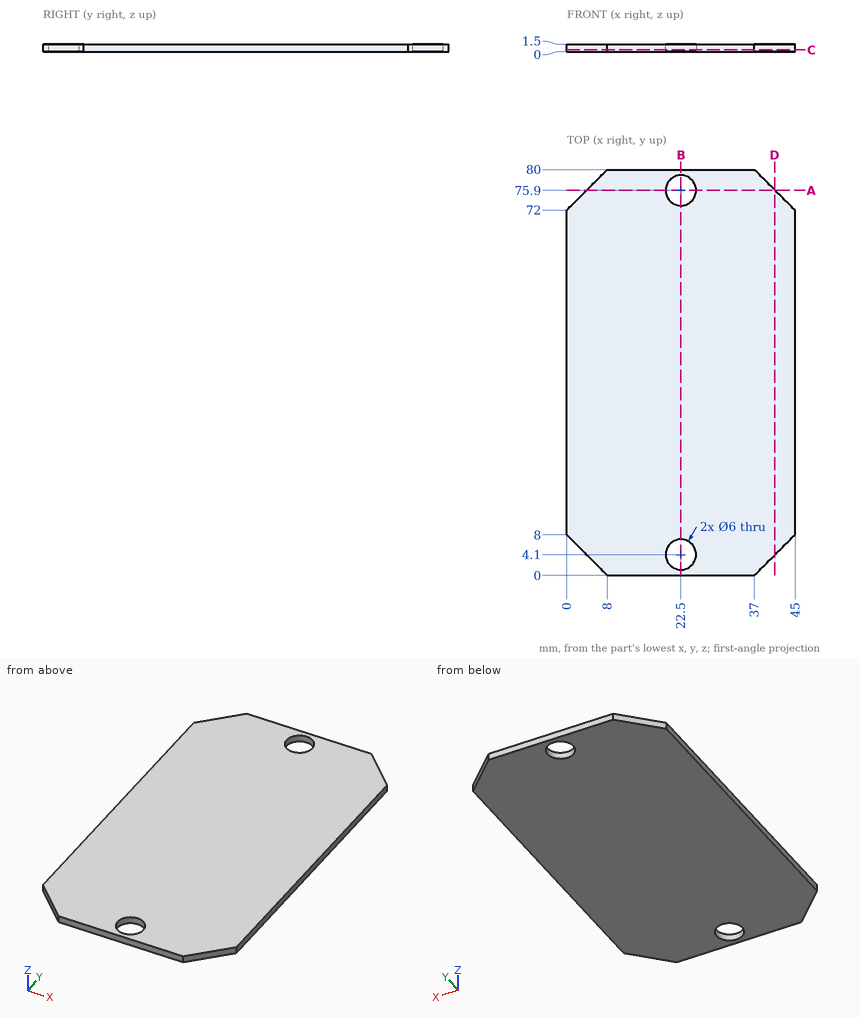
Answer from the drawing. Dimensions are ordinates in mm from the lowest x, y and z of the part. Round coordinates to 2 decimals unless told otherwise and drop trailing zeros. Order: outer loops, then holes, each group sorted by start corner. A loop starts at its lowest first (then second) coordinate and runs counter-clockwise, first axis right, second up.
1) The part is cut by section B-B on x = 22.5. Write down the section's boundary in (y, z).
2) Straight lines are drawn through the part: L1, parallel to Y at x = 22.5, z = 1.1; L2, parallel to Y at x = 20.5, z = 0.5; L3, parallel to X at y = 76.5, z = 0.7. For each, find the intervals that lie inside material, in ascending order.
3) The part is cut by section D-D on x = 41. Write down the section's boundary in (y, z), plus the area to 3 significant figures.
4) The part is cut by section C-C on z = 0.35. Write down the section's boundary in (x, y).
5) The part is cut by section A-A on y = 75.9. Write down the section's boundary in (x, z), plus the area to 3 significant figures.
Resolved:
1. outline: (0, 0) - (1.1, 0) - (1.1, 1.5) - (0, 1.5) - close; (7.1, 0) - (72.9, 0) - (72.9, 1.5) - (7.1, 1.5) - close; (78.9, 0) - (80, 0) - (80, 1.5) - (78.9, 1.5) - close
2. L1: y = 0 to 1.1, 7.1 to 72.9, 78.9 to 80
2. L2: y = 0 to 1.86, 6.34 to 73.66, 78.14 to 80
2. L3: x = 4.5 to 19.56, 25.44 to 40.5
3. outline: (4, 0) - (76, 0) - (76, 1.5) - (4, 1.5) - close
3. area: 108 mm2
4. outline: (0, 8) - (8, 0) - (37, 0) - (45, 8) - (45, 72) - (37, 80) - (8, 80) - (0, 72) - close; hole circle Ø6 at (22.5, 4.1); hole circle Ø6 at (22.5, 75.9)
5. outline: (3.9, 0) - (19.5, 0) - (19.5, 1.5) - (3.9, 1.5) - close; (25.5, 0) - (41.1, 0) - (41.1, 1.5) - (25.5, 1.5) - close
5. area: 46.8 mm2
